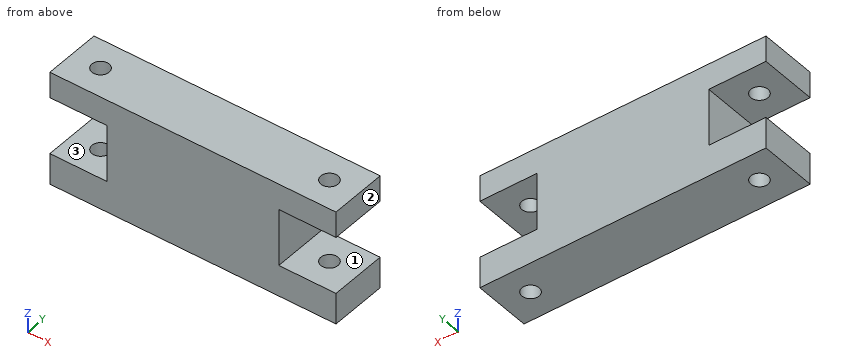
from build123d import *

# Parameters (mm, degrees)
SKETCH_1_W               = 100
SKETCH_1_H               = 20
EXTRUDE_1_DEPTH          = 40
CUT_EXTRUDE_1_DEPTH      = 68.082039325
SKETCH_4_R               = 3
CUT_EXTRUDE_2_DEPTH      = 59.695433862
MIRROR_3_COPY_1_SKETCH_R = 3
MIRROR_3_COPY_1_DEPTH    = 59.695433862


with BuildPart() as part:
    # 草图1 → 凸台-拉伸1 (new body)
    with BuildSketch(Plane.XY):
        Rectangle(SKETCH_1_W, SKETCH_1_H)
    extrude(amount=EXTRUDE_1_DEPTH)

    # 草图2 → 切除-拉伸1 (cut, through all)
    with BuildSketch(Plane(origin=(0, 10, 0), x_dir=(1, 0, 0), z_dir=(0, 1, 0))):
        Polygon((50, -10.928468285), (50, -20.928468285), (50, -30.928468285), (30, -30.928468285), (30, -10.928468285), align=None)
    cut_extrude_1 = extrude(amount=-CUT_EXTRUDE_1_DEPTH, mode=Mode.SUBTRACT)

    # 镜向1: 切除-拉伸1 across plane
    add(cut_extrude_1.mirror(Plane(origin=(0, 0, 0), x_dir=(0, 0, 1), z_dir=(1, 0, 0))), mode=Mode.SUBTRACT)

    # 草图4 → 切除-拉伸2 (cut, through all)
    with BuildSketch(Plane.XY.offset(10.928468285)):
        with Locations((40, 0)):
            Circle(SKETCH_4_R)
    cut_extrude_2 = extrude(amount=-CUT_EXTRUDE_2_DEPTH, mode=Mode.SUBTRACT)

    # 镜向2: 切除-拉伸2 across plane
    add(cut_extrude_2.mirror(Plane(origin=(0, 0, 0), x_dir=(0, 0, 1), z_dir=(1, 0, 0))), mode=Mode.SUBTRACT)

    # 镜向3: 切除-拉伸2 across plane
    add(cut_extrude_2.mirror(Plane.XY.offset(20)), mode=Mode.SUBTRACT)

    # 镜向3 copy 1 sketch → 镜向3 copy 1 (cut, through all)
    with BuildSketch(Plane(origin=(0, 0, 29.071531715), x_dir=(-1, 0, 0), z_dir=(0, 0, -1))):
        with Locations((40, 0)):
            Circle(MIRROR_3_COPY_1_SKETCH_R)
    extrude(amount=-MIRROR_3_COPY_1_DEPTH, mode=Mode.SUBTRACT)


solid = part.part
Here's how the part is built. I have some questions about the finished solid (model axes, mm). Face numbers are marked on the shaded views. A direction names the side the tool comes from. Round coordinates to 2 decimals unless told otherwise and drop trailing zeros. Loops run counter-clockwise (first coordinate to the right, second up) from the corner with the lowest first, then second, coordinate; pieces in that order, holes last. Notation, with made-up numbers: (39.5, 79) - (54.5, 79) arc R31 cw to (54.5, 117) - close; hole circle Ø11 at (7.5, 40.5). An arc over 180 degrees is marked (long way). One line per question, with ' | ' between items. Start each with the question number.
Q1. Please list where these lines run through material, in increasing order: line 1 (Z direction, x = -43, y = -8.5); line 2 (X direction, y = -1.5, z = 10); line 3 (Y direction, x = -40, z = 38). Write a range as [from, to].
Q2. For the marked faces 1, 2 and 3, which set-ups out of +Z, -Z, +X, -X, +Y, -Y let a thin tool reach every point of the face, with its end or its side?
Q3. I want a section at A-A (x = -40). Write out the boundary of the cut face in (y, z), then the cut area to 3 significant figures.
Q4. I want a section at C-C (z = 36.5). Write out the boundary of the cut face in (x, y).
Q5. I want a section at D-D (y = 5.5). Write out the boundary of the cut face in (x, z).
Q6. Will this pin go through, and if not, where does the flat tip stop? pin 1 (10 mm diameter, centred on y = -2.5, z = 18.5, fed in from +X).
Q7. I want a section at B-B (y = 0). Write out the boundary of the cut face in (x, z), then the cut area to 3 significant figures.
Response values:
1) line 1: z = [0, 10.93], [30.93, 40] | line 2: x = [-50, -42.6], [-37.4, 37.4], [42.6, 50] | line 3: y = [-10, -3], [3, 10]
2) face 1: +X, +Y, -Y | face 2: +Z, -Z, +X, +Y, -Y | face 3: -X, +Y, -Y
3) outline: (-10, 0) - (-3, 0) - (-3, 10.93) - (-10, 10.93) - close; (-10, 30.93) - (-3, 30.93) - (-3, 40) - (-10, 40) - close; (3, 0) - (10, 0) - (10, 10.93) - (3, 10.93) - close; (3, 30.93) - (10, 30.93) - (10, 40) - (3, 40) - close | area: 280 mm²
4) outline: (-50, -10) - (50, -10) - (50, 10) - (-50, 10) - close; hole circle Ø6 at (-40, 0); hole circle Ø6 at (40, 0)
5) outline: (-50, 0) - (50, 0) - (50, 10.93) - (30, 10.93) - (30, 30.93) - (50, 30.93) - (50, 40) - (-50, 40) - (-50, 30.93) - (-30, 30.93) - (-30, 10.93) - (-50, 10.93) - close
6) pin 1: stops at x = 30
7) outline: (-50, 0) - (-43, 0) - (-43, 10.93) - (-50, 10.93) - close; (-50, 30.93) - (-43, 30.93) - (-43, 40) - (-50, 40) - close; (-37, 0) - (37, 0) - (37, 10.93) - (30, 10.93) - (30, 30.93) - (37, 30.93) - (37, 40) - (-37, 40) - (-37, 30.93) - (-30, 30.93) - (-30, 10.93) - (-37, 10.93) - close; (43, 0) - (50, 0) - (50, 10.93) - (43, 10.93) - close; (43, 30.93) - (50, 30.93) - (50, 40) - (43, 40) - close | area: 2,960 mm²
